from build123d import *

# Parameters (mm, degrees)
F0_R     = 25.4
F1_DEPTH = 10.16
F2_R     = 1.27
F3_DEPTH = 5.08
F4_SIZE  = 5.08
F5_R     = 5.07999
F6_T     = 2.54


# Not quite as in the source:
# - a fillet or chamfer is up to 0.001 mm smaller than in the source, because OpenCascade refuses the exact size
# - a shell that OpenCascade refuses in one call is made with other operations: the cavity is built on its own and cut out


with BuildPart() as f1:
    # F0 (on Top) → F1 (new body)
    with BuildSketch(Plane.XY):
        Circle(F0_R)
    extrude(amount=F1_DEPTH)

    # F2 (on face) → F3 (cut)
    with BuildSketch(Plane.XY.offset(10.16)):
        Circle(F2_R)
    extrude(amount=-F3_DEPTH, mode=Mode.SUBTRACT)

    # F4
    f4_edges = [f1.edges().sort_by_distance(p)[0] for p in [
        (-25.4, 0, 10.16),
    ]]
    chamfer(f4_edges, length=F4_SIZE)

    # F5 (radius 5.08 in the source; OpenCascade refuses exactly that, so slightly less here)
    f5_edges = [f1.edges().sort_by_distance(p)[0] for p in [
        (-25.4, 0, 0),
    ]]
    fillet(f5_edges, radius=F5_R)

    # F6: shell of thickness 2.54, made by hand


with BuildPart() as f6_core1:
    # F6_t2: copy of F1
    add(f1.part)

    # the walls: a layer under each face that stays
    f6_faces = [f6_core1.faces().sort_by_distance(p)[0] for p in [
        (-25.4, 0, 5.079995),
        (-23.9121053774, 0, 1.4878946226),
        (-22.86, 0, 7.62),
        (-13.5466666667, -13.5466666667, 10.16),
        (-1.27, 0, 7.62),
        (0, 0, 5.08),
    ]]
    thicken(f6_faces, amount=-F6_T, mode=Mode.SUBTRACT)

    # F6_s3 → F6_t4 (revolve, cut)
    with BuildSketch(Plane.XZ):
        Polygon((1.2446, 5.1054), (3.81, 5.08), (3.81, 2.54), (1.27, 2.54), align=None)
    revolve(axis=Axis((0, 0, 5.08), (0, 0, 1)), mode=Mode.SUBTRACT)


with BuildPart() as f1_1:
    add(f1.part)

    # what is left inside the walls is the cavity
    f6_cavity = [f6_core1.part.solids().sort_by_distance(p)[0] for p in [
        (0, -6.773337, 0.0254),
    ]]
    add(f6_cavity, mode=Mode.SUBTRACT)


solid = f1_1.part
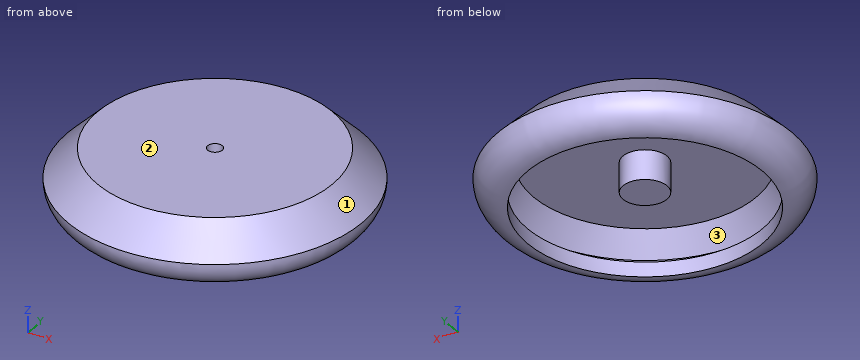
Work out the finished part from the listing and answer in its coordinate system (mm). Face numbers are marked on the shaded views. Coordinates: 2 decimals unless noted, no trailing zeros. Write each loop counter-clockwise with the first axis right and the second up, starting at its lowest first coordinate (ties: lowest second). Pieces come first, ordered by that corner, then holes. Notation, with made-up numbers: M 48,62 L 106,62 A26 cw 106,96 Z; hole C -25,85.5 d5. An arc over 180 degrees is marked long. Use one line per item in the form item = value. Start each with the question number.
1. The part is cut by section D-D (z = 1.75). Give the vertices of the cut face in (x, y).
2. The part is cut by section B-B (z = 5.75). Give the vertices of the cut face in (x, y), plus the area to 3 significant figures.
3. Each of these flat-tipped pins is pushed along its axis until it touches: P1, Ø1.5, axis at x = 6.5, z = 3.5, coming from the -Y side; P2, Ø19.5, axis at x = -5, y = 4, coming from the -Z side; P3, Ø2, axis at x = 0, y = 0.5, coming from the +Z side; P4, Ø6, axis at x = 10, z = 3, coming from the -Y side. Where does it stop, or does it pass through?
4. Straight lines are drawn through the part: probe 1 along X at (y, z) = (14, 1.75); probe 2 along Y at (x, z) = (0, 1.65); probe 3 along Z at (x, y) = (-16, -8.5). For each, find the intervals that lie inside material, in ascending order. Write a range as from..to.
5. The mould has two halves that part along X. Classify the marked faces 1, 2 and 3: released by +X, released by -X, zero draft, split by the parting line, or undercut.
Evaluation:
q1.outline = C 0,0 d48.31; hole C 0,0 d40.64
q2.outline = C 0,0 d49.46; C 0,0 d7.62; hole C 0,0 d42.28; hole C 0,0 d2.54
q2.area = 558 mm^2
q3.P1 = -24.58
q3.P2 = 2.54
q3.P3 = 10.16
q3.P4 = -24.27
q4.probe_1 = -19.69..-14.73, 14.73..19.69
q4.probe_2 = -24.07..-20.32, 20.32..24.07
q4.probe_3 = 7.62..10.16
q5.face_1 = split by the parting line
q5.face_2 = zero draft
q5.face_3 = undercut
